Source: CAD feature listing. Evaluate the final solid. Frame: model axes, mm. A direction names the side the tool comes from. Give positions to 0.01 mm unless a question says otherwise; leave off trailing zeros. Order: outer loops, then holes, each group sorted by start corner. A loop starts at its lowest first (then second) coordinate and runs counter-clockwise, first axis right, second up. Notation, with made-up numbers: M 71,36.25 L 127,36.25 A21 ccw 127,75.25 Z; hole C 25.5,-39.75 d9. An arc over 180 degrees is marked long. Return JSON: item names as keys, results as strings.
from build123d import *

# Parameters (mm, degrees)
F0_W      = 70
F0_H      = 50
F1_DEPTH  = 1.5
F2_W      = 46
F2_H      = 46
F3_DEPTH  = 12.5
F2_W_2    = 5
F2_H_2    = 10
F4_DEPTH  = 10
F5_W      = 51
F5_H      = 46
F6_DEPTH  = 9
F7_W      = 50
F7_H      = 3
F7_H_2    = 1.5
F7_H_3    = 12.5
F8_DEPTH  = 31.8
F9_W      = 31.8
F9_H      = 40
F9_W_2    = 15
F10_DEPTH = 1.5
F12_DEPTH = 3


with BuildPart() as f1:
    # F0 (on Top) → F1 (new body)
    with BuildSketch(Plane.XY):
        with Locations((35, 25)):
            Rectangle(F0_W, F0_H)
    extrude(amount=F1_DEPTH)

    # F2 (on face) → F3 (join)
    with BuildSketch(Plane(origin=(0, 0, 0), x_dir=(1, 0, 0), z_dir=(0, 0, -1))):
        with Locations((43, -25)):
            Rectangle(F2_W, F2_H)
    extrude(amount=F3_DEPTH)

    # F2 (on face) → F4 (join)
    with BuildSketch(Plane(origin=(0, 0, 0), x_dir=(1, 0, 0), z_dir=(0, 0, -1))):
        with Locations((5.7, -25)):
            Rectangle(F2_W_2, F2_H_2)
    extrude(amount=F4_DEPTH)

    # F5 (on face) → F6 (join)
    with BuildSketch(Plane.XY.offset(1.5)):
        with Locations((40.5, 25)):
            Rectangle(F5_W, F5_H)
    extrude(amount=F6_DEPTH)

    # F7 (on face) → F8 (join)
    with BuildSketch(Plane(origin=(0, 0, 0), x_dir=(0, -1, 0), z_dir=(-1, 0, 0))):
        with Locations((-25, 3)):
            Rectangle(F7_W, F7_H)
        with Locations((-25, 0.75)):
            Rectangle(F7_W, F7_H_2)
        with Locations((-25, -6.25)):
            Rectangle(F7_W, F7_H_3)
    extrude(amount=F8_DEPTH)

    # F9 (on face) → F10 (join)
    with BuildSketch(Plane.XY.offset(4.5)):
        with Locations((-15.9, 25)):
            Rectangle(F9_W, F9_H)
        with Locations((7.5, 25)):
            Rectangle(F9_W_2, F9_H)
    extrude(amount=F10_DEPTH)

    # F11 (on face) → F12 (cut)
    with BuildSketch(Plane(origin=(-31.8, 0, 0), x_dir=(0, -1, 0), z_dir=(-1, 0, 0))):
        Polygon((-5, 4.5), (-45, 4.5), (-50, 4.5), (-50, -12.5), (0, -12.5), (0, 4.5), align=None)
    extrude(amount=-F12_DEPTH, mode=Mode.SUBTRACT)


solid = f1.part
1. Draft query along Z for faces 1 (the face through (0, 25, 3)), 2 (the face through (-14, 48, 4.5)), 3 (the face through (-5, 50, -5)), 4 (the face through (14, 25, 1.5)). Return one class per face: pulls with the +Z half, pulls with the -Z half, needs draft (parallel to the pull), parting line crosses it, or undercut.
Evaluation:
{"face 1": "undercut", "face 2": "pulls with the +Z half", "face 3": "needs draft", "face 4": "undercut"}
2. Ray query, probe 1 along X at (y, z) = (21.5, 3); probe 2 along X at (y, z) = (26, -3.5); probe 3 along X at (y, z) = (31.5, -0.75). Return the intervals inside material, ascending.
Evaluation:
{"probe 1": "x = -28.8 to 0, 15 to 66", "probe 2": "x = -28.8 to 0, 3.2 to 8.2, 20 to 66", "probe 3": "x = -28.8 to 0, 20 to 66"}
3. Set-up query: faces 5 (the face through (6, 30, -5)), 6 (the face through (20, 25, -6)), 7 (the face through (66, 25, 6)). Return all of +Z, -Z, +X, -X, +Y, -Y with unobstructed straight access to the full face (end or side cutting, diameter ignored); none if empty.
Evaluation:
{"face 5": "-Z, +Y", "face 6": "-Z, +Y, -Y", "face 7": "+Z, +X, +Y, -Y"}
4. Section query B-B (z = -7.5). Return loops of the section in (x, y), then the cut area to 3 significant figures.
Evaluation:
{"outline": "M -28.8,0 L 0,0 L 0,50 L -28.8,50 Z; M 3.2,20 L 8.2,20 L 8.2,30 L 3.2,30 Z; M 20,2 L 66,2 L 66,48 L 20,48 Z", "area": "3,610 mm^2"}
5. First-contact query: pin 1 (5.5 mm diameter, centred on x = -17.5, y = 46.5, fed in from +Z); pin 2 (1 mm diameter, centred on x = 9, z = 4.5, fed in from -Y); pin 3 (1.2 mm diameter, centred on x = 1, z = 5.5, fed in from +Y). Flat tips, straight axial feed; report the tip coordinate or a pass-through.
Evaluation:
{"pin 1": "stops at z = 6", "pin 2": "stops at y = 5", "pin 3": "stops at y = 45"}
6. Section query C-C (y = 23.5). Return loops of the section in (x, z).
Evaluation:
{"outline": "M -31.8,4.5 L -28.8,4.5 L -28.8,-12.5 L 0,-12.5 L 0,0 L 3.2,0 L 3.2,-10 L 8.2,-10 L 8.2,0 L 20,0 L 20,-12.5 L 66,-12.5 L 66,0 L 70,0 L 70,1.5 L 66,1.5 L 66,10.5 L 15,10.5 L 15,6 L -31.8,6 Z; hole M 0,1.5 L 15,1.5 L 15,4.5 L 0,4.5 Z"}
7. Section query D-D (z = 2.5). Return loops of the section in (x, y), then the cut area to 3 significant figures.
Evaluation:
{"outline": "M -28.8,0 L 0,0 L 0,50 L -28.8,50 Z; M 15,2 L 66,2 L 66,48 L 15,48 Z", "area": "3,790 mm^2"}
8. Section query A-A (x = 1). Return loops of the section in (y, z), then the cut area to 3 significant figures.
Evaluation:
{"outline": "M 0,0 L 50,0 L 50,1.5 L 0,1.5 Z; M 5,4.5 L 45,4.5 L 45,6 L 5,6 Z", "area": "135 mm^2"}
